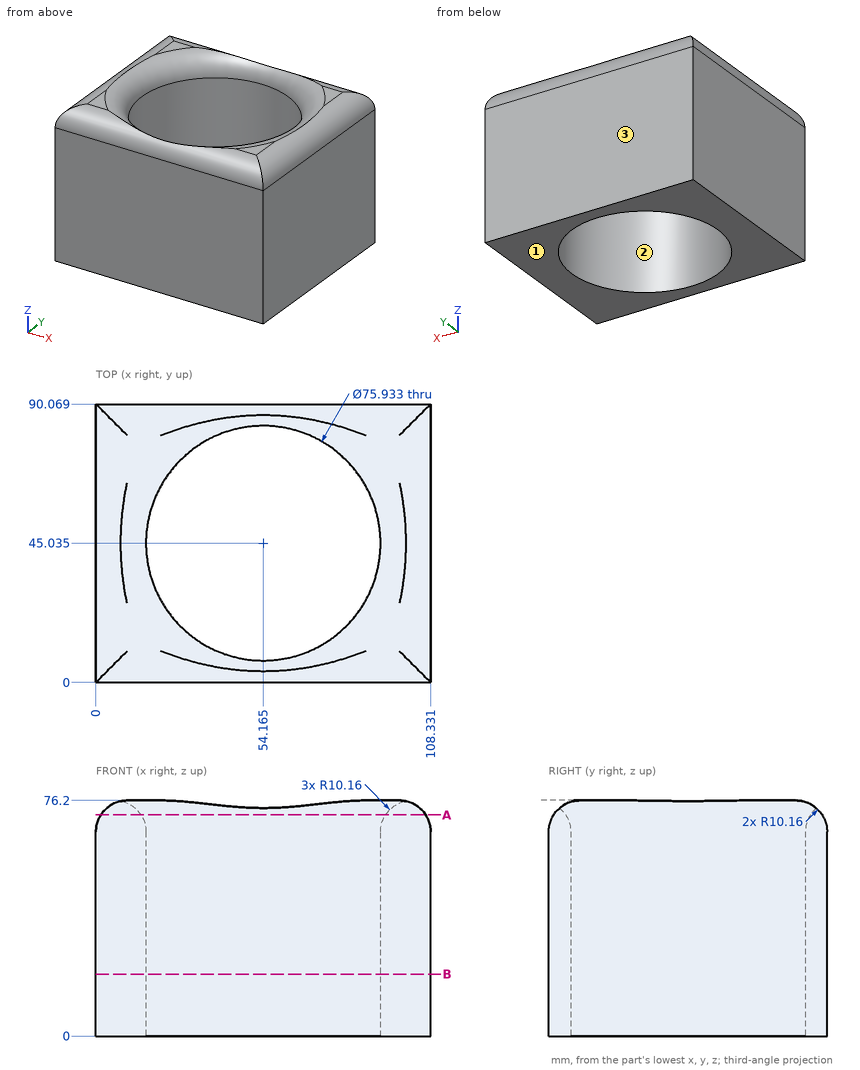
The drawing under review shows one solid part. Ordinate dimensions are in mm from its lowest x, y, z. Give positions to 0.01 mm unless a question says otherwise; leave off trailing zeros. Write each loop counter-clockwise with the first axis right and the second up, starting at its lowest first coordinate (ties: lowest second). Pieces come first, ordered by that corner, then holes. Notation, with made-up numbers: M -25,60 L 0,60 A13 ccw 0,71 Z; hole C 86,-27 d5. An arc over 180 degrees is marked long. Write each question's results on one line, items separated by ' | '. Start each with the question number.
1. Insertion check: pin 1 Ø10 at (x, y) = (24, 65) entering from +Z. The pin has a flat end and moves straight along its axis. Give the tip position at first contact, or say it passes through.
2. We need section B-B (z = 20). Write out the cut boundary in (x, y) (1 decimal).
3. For probe 1 along Y at (x, z) = (55.5, 52); probe 2 along X at (y, z) = (46.5, 26); probe 3 along X at (y, z) = (13, 61) (1 decimal), list the stretches that pass through material, from the lowest coordinate up. Write a range as [from, to].
4. Mouldability with a two-part tool opening along Y and no side actions: class the marked faces 1, 2 and 3 as released by +Y, released by -Y, zero draft, split by the parting line, or undercut.
5. We need section A-A (z = 71.5). Write out the cut boundary in (x, y) (1 decimal), and give its area (3 significant figures).
Results found:
1) pin 1: stops at z = 73.45
2) outline: M 0,0 L 108.3,0 L 108.3,90.1 L 0,90.1 Z; hole C 54.2,45 d75.9
3) probe 1: y = [0, 7.09], [82.98, 90.07] | probe 2: x = [0, 16.23], [92.1, 108.33] | probe 3: x = [0, 33.8], [74.5, 108.3]
4) face 1: zero draft | face 2: undercut | face 3: released by +Y
5) outline: M 1.6,1.6 L 106.7,1.6 L 106.7,88.5 L 1.6,88.5 Z; hole C 54.2,45 d79.1 | area: 4,220 mm^2
